Part model, mm, in its own coordinate system. A direction names the side the tool comes from. Round coordinates to 2 decimals unless told otherwise and drop trailing zeros. Write each loop counter-clockwise with the first axis right and the second up, starting at its lowest first coordinate (ties: lowest second). Pieces come first, ordered by that corner, then holes.
```python
from build123d import *

# Parameters (mm, degrees)
CHAMFER_1_SIZE           = 0.3
SKETCH_2_R               = 2.1
CUT_EXTRUDE_1_DEPTH      = 58.493477891
PATTERN_CIRCULAR_1_COUNT = 4
HOLE_WIZARD_M4_1_D       = 3.3
PATTERN_CIRCULAR_2_COUNT = 8


with BuildPart() as part:
    # 草图1 → 旋转1 (revolve)
    with BuildSketch(Plane.XY, mode=Mode.PRIVATE) as revolve_1_sk:
        Polygon((0, 28.5), (0, 21.05), (39.5, 21.05), (39.5, 13.15), (41, 13.15), (41, 22.25), (16, 22.25), (16, 22.5), (9, 22.5), (9, 23.25), (4, 23.25), (4, 28.5), align=None)
    revolve(revolve_1_sk.sketch.rotate(Axis((0, 0, 0), (1, 0, 0)), 90), axis=Axis((0, 0, 0), (1, 0, 0)))

    # 倒角1
    chamfer_1_edges = [part.edges().sort_by_distance(p)[0] for p in [
        (41, 0, -13.15),
        (41, 0, -22.25),
        (4, 0, -28.5),
        (0, 0, -28.5),
        (39.5, 0, -13.15),
    ]]
    chamfer(chamfer_1_edges, length=CHAMFER_1_SIZE)

    # 草图2 → 切除-拉伸1 (cut, symmetric)
    with BuildSketch(Plane(origin=(41, 0, 0), x_dir=(0, 0, -1), z_dir=(1, 0, 0))):
        with Locations((5.697442703, 16.546575073)):
            Circle(SKETCH_2_R)
    cut_extrude_1 = extrude(amount=CUT_EXTRUDE_1_DEPTH, both=True, mode=Mode.SUBTRACT)

    # 阵列(圆周)1: 切除-拉伸1 ×4 about axis
    pattern_circular_1_axis = Axis((0, 0, 0), (1, 0, 0))
    for i in range(1, PATTERN_CIRCULAR_1_COUNT):
        add(cut_extrude_1.rotate(pattern_circular_1_axis, i * 360 / PATTERN_CIRCULAR_1_COUNT), mode=Mode.SUBTRACT)

    # M4 螺纹孔1 (through all)
    with Locations(Plane.ZY):
        with Locations((-9.567085809, -23.096988313)):
            hole_wizard_m4_1 = Hole(HOLE_WIZARD_M4_1_D / 2)

    # 阵列(圆周)2: M4 螺纹孔1 ×8 about axis
    pattern_circular_2_axis = Axis((0, 0, 0), (1, 0, 0))
    for i in range(1, PATTERN_CIRCULAR_2_COUNT):
        add(hole_wizard_m4_1.rotate(pattern_circular_2_axis, i * 360 / PATTERN_CIRCULAR_2_COUNT), mode=Mode.SUBTRACT)


solid = part.part
```
Q1. Which spindle directions (+Z, -Z, +X, -X, +Y, -Y) get a long thin tool onto all of the face, cutting with end or side? Do faces 4 (the cylindrical face through (2.028, -9.209, 24.708)), 5 (the cylindrical face through (6.465, -6.984, 22.176)), 6 (the flat face through (39.5, 0, 14)). Say none if no direction does.
Values follow:
face 4: +X, -X
face 5: +X
face 6: -X
Q2. Mould opens along Y. For faces 1 (the cylindrical face through (2.028, -24.708, -9.209)), 2 (the flat face through (4, 21, 11)), 3 (the cylindrical face through (28.177, -15.038, -16.399)) say: +Y half, -Y half, draft (parallel to the pull), parting line (faces both ways), or undercut.
Values follow:
face 1: undercut
face 2: draft
face 3: parting line
Q3. Cut at C-C on x = 19. Write the cut outline in (y, z), plus the area to 3 significant figures.
Values follow:
outline: circle Ø44.5 at (0, 0); hole circle Ø42.1 at (0, 0)
area: 163 mm2
Q4. Wall check: L1, parallel to Y at x = 3, z = -9; L2, parallel to X at y = -12.5, z = 24; L3, parallel to Z at x = 28, y = -5. Give the ranges that are in metal, low to high.
Values follow:
L1: y = -27.04 to -24.65, -21.55 to -19.03, 19.03 to 21.55, 24.65 to 27.04
L2: x = 0 to 4
L3: z = -21.68 to -20.45, 20.45 to 21.68
Q5. Cut at D-D on z = 7. State how many separate pieces and enclosed holes the cut face has, plus the area to 3 significant figures.
Values follow:
separate pieces: 3
enclosed holes: 0
area: 191 mm2
Q6. Drop flat-ended pins along their axis: pin 1 (5 mm diameter, centred on x = 4.5, y = -18.5, fed in from +Z); pin 2 (2 mm diameter, centred on x = 15, z = 10.5, fed in from +Y); pin 3 (12 mm diameter, centred on x = 34, y = 16.5, fed in from +Z). Give the stop position or say it passes through.
Values follow:
pin 1: stops at z = 23.5
pin 2: stops at y = 20.4
pin 3: stops at z = 19.62
